```python
from build123d import *

# Parameters (mm, degrees)
BOSS_EXTRUDE1_DEPTH                   = 12.7
TAP_DRILL_FOR_M6X1_0_TAP1_D           = 5
TAP_DRILL_FOR_M6X1_0_TAP1_CSINK_D     = 5.05
TAP_DRILL_FOR_M6X1_0_TAP1_CSINK_ANGLE = 90
M6_CLEARANCE_HOLE1_D                  = 6.6
M6_CLEARANCE_HOLE1_CSINK_D            = 6.65
M6_CLEARANCE_HOLE1_CSINK_ANGLE        = 90
FILLET1_R                             = 1


with BuildPart() as part:
    # Sketch1 → Boss-Extrude1 (new body)
    with BuildSketch(Plane.XY):
        with BuildLine():
            Line((-26, 0), (26, 0))
            Line((26, 0), (26, 6))
            Line((26, 6), (11, 6))
            ThreePointArc((11, 6), (10.408351378, 10.95046998), (7.5, 15))
            Line((7.5, 15), (-7.5, 15))
            ThreePointArc((-7.5, 15), (-10.408351378, 10.95046998), (-11, 6))
            Line((-11, 6), (-26, 6))
            Line((-26, 6), (-26, 0))
        make_face()
    extrude(amount=-BOSS_EXTRUDE1_DEPTH)

    # Tap Drill for M6x1.0 Tap1 (through all)
    with Locations(Plane(origin=(0, 10, 0), x_dir=(1, 0, 0), z_dir=(0, 0, 1))):
        with Locations((0, 0)):
            CounterSinkHole(TAP_DRILL_FOR_M6X1_0_TAP1_D / 2, TAP_DRILL_FOR_M6X1_0_TAP1_CSINK_D / 2, counter_sink_angle=TAP_DRILL_FOR_M6X1_0_TAP1_CSINK_ANGLE)

    # M6 Clearance Hole1 (through all)
    with Locations(Plane(origin=(-20, 0, -6.35), x_dir=(-1, 0, 0), z_dir=(0, -1, 0))):
        with Locations((0, 0), (-40, 0)):
            CounterSinkHole(M6_CLEARANCE_HOLE1_D / 2, M6_CLEARANCE_HOLE1_CSINK_D / 2, counter_sink_angle=M6_CLEARANCE_HOLE1_CSINK_ANGLE)

    # Fillet1
    fillet1_edges = [part.edges().sort_by_distance(p)[0] for p in [
        (-26, 6, -6.35),
        (26, 6, -6.35),
        (11, 6, -6.35),
        (7.5, 15, -6.35),
        (-7.5, 15, -6.35),
        (-11, 6, -6.35),
    ]]
    fillet(fillet1_edges, radius=FILLET1_R)


solid = part.part
```
Check sheet for the modelled part. Datum: model origin and axes. Units: mm. A direction names the side the tool comes from. Round coordinates to 2 decimals unless told otherwise and drop trailing zeros. Order: outer loops, then holes, each group sorted by start corner. A loop starts at its lowest first (then second) coordinate and runs counter-clockwise, first axis right, second up. Notation, with made-up numbers: (-32, 18) -> (-13, 18) arc R12 ccw to (-13, 32) -> close; hole circle Ø7 at (73.5, -1.5). An arc over 180 degrees is marked (long way). One line per item, written item: value. Start each with the question number.
Q1. Cross-section at D-D (y = 2.5). Record the boundary of the cut face in (x, z).
Q2. Mould release check, pull along Y, two halves, no side actions. Record for faces 1 (the face through (0, 0, -6)), 2 (the face through (0.54, 7.56, -6.45)), 3 (the face through (-26, 3, -6)), 4 (the face through (25.699, 5.715, -6.439)): pulls with the +Y half, pulls with the -Y half, needs draft (parallel to the pull), parting line crosses it, or undercut.
Q3. Gauge pin test, flat ends, axial feed: pin 1 Ø6 at (x, z) = (-20, -6.35) entering from +Y; pin 2 Ø4 at (x, z) = (19, -9.5) entering from +Y. Record the tip position at first contact, or that the pin passes through.
Q4. Cross-section at A-A (x = 0). Record the boundary of the cut face in (y, z) (3 decimals).
Q5. Cross-section at C-C (z = -6.35). Record the boundary of the cut face in (x, y) (3 decimals).
Q6. Cross-section at B-B (y = 10). Record the boundary of the cut face in (x, z) (3 decimals).
Q7. Set-up check for faces 5 (the face through (-16, 6, -6)), 6 (the face through (16, 6, -6)), 7 (the face through (0, 6, 0)): record each of +Z, -Z, +X, -X, +Y, -Y from which the full face is reachable in a straight line by a thin tool's end or side.
Q8. Thickness scan on line 1 (Z direction, x = -20, y = 3.25); line 2 (Y direction, x = 0, z = -3.5); line 3 (X direction, y = 3, z = -4.5). Record the ranges inside material, lowest first.
Completed:
1. outline: (-26, -12.7) -> (26, -12.7) -> (26, 0) -> (-26, 0) -> close; hole circle Ø6.6 at (-20, -6.35); hole circle Ø6.6 at (20, -6.35)
2. face 1: pulls with the -Y half
2. face 2: undercut
2. face 3: needs draft
2. face 4: pulls with the +Y half
3. pin 1: passes through
3. pin 2: stops at y = 6
4. outline: (0, -12.7) -> (7.5, -12.7) -> (7.5, -0.025) -> (7.475, 0) -> (0, 0) -> close; (12.5, -12.7) -> (15, -12.7) -> (15, 0) -> (12.525, 0) -> (12.5, -0.025) -> close
5. outline: (-26, 0) -> (-23.325, 0) -> (-23.3, 0.025) -> (-23.3, 6) -> (-25, 6) arc R1 ccw to (-26, 5) -> close; (-16.7, 0.025) -> (-16.675, 0) -> (16.675, 0) -> (16.7, 0.025) -> (16.7, 6) -> (12.083, 6) arc R1 cw to (11.084, 7.03) arc R10 ccw to (7.797, 14.742) arc R1 ccw to (7.126, 15) -> (-7.126, 15) arc R1 ccw to (-7.797, 14.742) arc R10 ccw to (-11.084, 7.03) arc R1 cw to (-12.083, 6) -> (-16.7, 6) -> close; (23.3, 0.025) -> (23.325, 0) -> (26, 0) -> (26, 5) arc R1 ccw to (25, 6) -> (23.3, 6) -> close; hole circle Ø5 at (0, 10)
6. outline: (-10.724, -12.7) -> (-2.5, -12.7) -> (-2.5, -0.025) -> (-2.525, 0) -> (-10.724, 0) -> close; (2.5, -12.7) -> (10.724, -12.7) -> (10.724, 0) -> (2.525, 0) -> (2.5, -0.025) -> close
7. face 5: +Z, -Z, -X, +Y
7. face 6: +Z, -Z, +X, +Y
7. face 7: +Z, +X, -X, +Y, -Y
8. line 1: z = -12.7 to -9.65, -3.05 to 0
8. line 2: y = 0 to 7.5, 12.5 to 15
8. line 3: x = -26 to -22.73, -17.27 to 17.27, 22.73 to 26
